Model file for the job. Use its own axes, mm. A direction names the side the tool comes from. Round coordinates to 2 decimals unless told otherwise and drop trailing zeros. Order: outer loops, then holes, each group sorted by start corner. A loop starts at its lowest first (then second) coordinate and runs counter-clockwise, first axis right, second up. Notation, with made-up numbers: (63.5, 30) - (108.5, 30) arc R16 ccw to (108.5, 52) - close; hole circle Ø2 at (-35, -24.75). An arc over 180 degrees is marked (long way). Write item = value, one per line.
```python
from build123d import *

# Parameters (mm, degrees)
BOSS_EXTRUDE1_DEPTH          = 476.25
F_10_0_1935_DIAMETER_HOLE1_D = 4.9149
F_10_0_1935_DIAMETER_HOLE2_D = 4.9149


with BuildPart() as part:
    # Sketch2 → Boss-Extrude1 (new body)
    with BuildSketch(Plane.XY):
        Polygon((0, 0), (0, 31.75), (1.5875, 31.75), (1.5875, 1.5875), (31.75, 1.5875), (31.75, 0), align=None)
    extrude(amount=BOSS_EXTRUDE1_DEPTH)

    # #10 (0.1935) Diameter Hole1 (through all)
    with Locations(Plane.ZY):
        with Locations((95.25, 15.875), (381, 15.875)):
            Hole(F_10_0_1935_DIAMETER_HOLE1_D / 2)

    # #10 (0.1935) Diameter Hole2 (through all)
    with Locations(Plane(origin=(0, 0, 0), x_dir=(-1, 0, 0), z_dir=(0, -1, 0))):
        with Locations((-15.875, -95.25), (-15.875, -381)):
            Hole(F_10_0_1935_DIAMETER_HOLE2_D / 2)


solid = part.part
```
1) Flat gauge pins, fed straight in: pin 1 Ø8 at (x, z) = (15.875, 381) entering from +Y; pin 2 Ø12 at (y, z) = (10, 108) entering from +X. Where does each tip first touch, or does it go through?
Conclusion:
pin_1 = 1.59
pin_2 = 1.59
2) 3-axis set-ups, long thin cutter, end or side, ignore diameter. For faces 1 (the face through (16, 1.588, 235)), 2 (the face through (9, 1, 476.25)): which of +Z, -Z, +X, -X, +Y, -Y reach the whole face in a straight line?
Conclusion:
face_1 = +Z, -Z, +X, +Y
face_2 = +Z, +X, -X, +Y, -Y
3) Cut at A-A (z = 118). Write the cut outline in (x, y), and give its area (3 significant figures).
Conclusion:
outline = (0, 0) - (31.75, 0) - (31.75, 1.59) - (1.59, 1.59) - (1.59, 31.75) - (0, 31.75) - close
area = 98.3 mm^2
4) Wall check: line 1 along Y through (x, z) = (0.4, 381); line 2 along X through (y, z) = (25, 193). Give the ranges that are in metal, low to high.
Conclusion:
line_1 = 0 to 13.42, 18.33 to 31.75
line_2 = 0 to 1.59
5) Cut at B-B (y = 7). Write the cut outline in (x, z).
Conclusion:
outline = (0, 0) - (1.59, 0) - (1.59, 476.25) - (0, 476.25) - close
